Geometry: final body of the model. Coordinates: model frame, mm. Face numbers are marked on the shaded views. A direction names the side the tool comes from. Give positions to 0.01 mm unless a question says otherwise; leave off trailing zeros. Write each loop counter-clockwise with the first axis right and the second up, starting at its lowest first coordinate (ties: lowest second). Pieces come first, ordered by that corner, then holes. Notation, with made-up numbers: M 60.5,54 L 71.5,54 A8 cw 71.5,69 Z; hole C 36.25,-33 d8. An arc over 180 degrees is marked long. Answer as a JSON object with one key per item and string values.
from build123d import *

# Parameters (mm, degrees)
SKETCH1_R           = 50.8
SKETCH1_W           = 38.0365
SKETCH1_H           = 12.7508
BOSS_EXTRUDE1_DEPTH = 5.6642
SKETCH1_3_R         = 50.8
SKETCH1_3_W         = 38.0365
SKETCH1_3_H         = 12.7508
SKETCH1_3_R_2       = 3.71475
BOSS_EXTRUDE2_DEPTH = 5.715
BOSS_EXTRUDE3_DEPTH = 15.875
CUT_EXTRUDE1_DEPTH  = 22.5392


with BuildPart() as part:
    # Sketch1 → Boss-Extrude1 (new body)
    with BuildSketch(Plane(origin=(0, 0, 0), x_dir=(1, 0, 0), z_dir=(0, 1, 0))):
        Circle(SKETCH1_R)
        Rectangle(SKETCH1_W, SKETCH1_H, mode=Mode.SUBTRACT)
    extrude(amount=BOSS_EXTRUDE1_DEPTH)

    # Sketch1_3 → Boss-Extrude2 (add)
    with BuildSketch(Plane(origin=(0, 0, 0), x_dir=(1, 0, 0), z_dir=(0, 1, 0))):
        Circle(SKETCH1_3_R)
        Rectangle(SKETCH1_3_W, SKETCH1_3_H, mode=Mode.SUBTRACT)
        Rectangle(SKETCH1_3_W, SKETCH1_3_H)
        Circle(SKETCH1_3_R_2, mode=Mode.SUBTRACT)
    extrude(amount=-BOSS_EXTRUDE2_DEPTH)

    # Sketch2 → Boss-Extrude3 (add, symmetric)
    with BuildSketch(Plane(origin=(0, 0, 0), x_dir=(1, 0, 0), z_dir=(0, 1, 0))):
        with BuildLine():
            Line((-32.174984, 35.112833), (-34.319983, 37.453689))
            ThreePointArc((-34.319983, 37.453689), (0, 50.8), (34.319983, 37.453689))
            Line((34.319983, 37.453689), (32.174984, 35.112833))
            ThreePointArc((32.174984, 35.112833), (0, 47.625), (-32.174984, 35.112833))
        make_face()
        with BuildLine():
            Line((-25.588894, -40.166518), (-27.29482, -42.844285))
            ThreePointArc((-27.29482, -42.844285), (0, -50.8), (27.29482, -42.844285))
            Line((27.29482, -42.844285), (25.588894, -40.166518))
            ThreePointArc((25.588894, -40.166518), (0, -47.625), (-25.588894, -40.166518))
        make_face()
    extrude(amount=BOSS_EXTRUDE3_DEPTH, both=True)

    # Sketch3 → Cut-Extrude1 (cut, through all)
    with BuildSketch(Plane(origin=(0, 5.6642, 0), x_dir=(1, 0, 0), z_dir=(0, 1, 0))):
        with BuildLine():
            Line((-31.75, 17.8054), (31.75, 17.8054))
            ThreePointArc((31.75, 17.8054), (0, 33.0454), (-31.75, 17.8054))
        make_face()
        with BuildLine():
            Line((-31.75, -17.8054), (31.75, -17.8054))
            ThreePointArc((31.75, -17.8054), (0, -33.0454), (-31.75, -17.8054))
        make_face()
    extrude(amount=-CUT_EXTRUDE1_DEPTH, mode=Mode.SUBTRACT)


solid = part.part
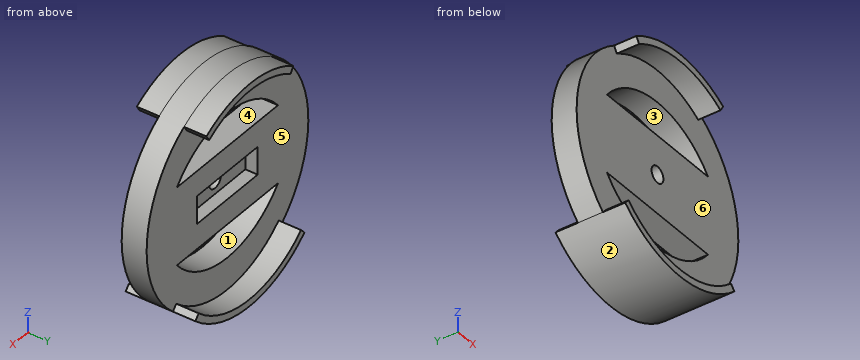
1) Set-up query: the marked faces 4, 5 and 6. Return all of +Z, -Z, +X, -X, +Y, -Y with unobstructed straight access to the full face (end or side cutting, diameter ignored); none if empty.
Geometry check:
{"face 4": "+Y, -Y", "face 5": "+Y", "face 6": "-Y"}
2) Cut plane A-A on y = 7.5. Return loops of the section in (x, z) (3 decimals).
Geometry check:
{"outline": "M -34.32,-37.454 A50.8 ccw 34.32,-37.454 L 32.175,-35.113 A47.625 cw -32.175,-35.113 Z; M -27.295,42.844 L -25.589,40.167 A47.625 cw 25.589,40.167 L 27.295,42.844 A50.8 ccw Z"}
3) Line query: line 1 (X direction, y = -2.2, z = 0); line 2 (Y direction, x = 11.5, z = 3.5) (3 decimals); line 3 (Y direction, x = 21, z = -30) (3 decimals). Output: solid intervals per line, ascending. Write a range as from..to.
Geometry check:
{"line 1": "x = -50.8..-3.71, 3.71..50.8", "line 2": "y = -5.715..0", "line 3": "y = -5.715..5.664"}
4) Cut plane D-D on y = -3. Return loops of the section in (x, z), and give its area (3 significant figures).
Geometry check:
{"outline": "M -34.32,-37.45 A50.8 ccw 34.32,-37.45 A50.8 ccw long Z; hole M -31.75,-17.81 A40.69 ccw 31.75,-17.81 Z; hole M -31.75,17.81 L 31.75,17.81 A40.69 ccw Z; hole C 0,0 d7.43", "area": "6,720 mm2"}
5) Cut plane B-B on z = -23.5. Return loops of the section in (x, y) (3 decimals).
Geometry check:
{"outline": "M -45.038,-5.715 L -26.187,-5.715 L -26.187,5.664 L -45.038,5.664 Z; M 26.187,-5.715 L 45.038,-5.715 L 45.038,5.664 L 26.187,5.664 Z"}
6) Contact query for flat-ended pins moving along their axis: P1, Ø1.5, axis at x = -35.5, y = 8.5, coming from the -Z side; P2, Ø2, axis at x = 31.5, y = 2, coming from the +Z side (3 decimals); P3, Ø12.5, axis at x = -11, y = 2, coming from the -Z side; P4, Ø1.7, axis at x = -6.5, y = 2.5, coming from the -Z side. Output: stop coordinate, or through.
Geometry check:
{"P1": "passes through", "P2": "stops at z = 40.625", "P3": "stops at z = -50.58", "P4": "stops at z = -50.48"}
7) Cut plane C-C on x = -17.5. Return loops of the section in (y, z) (3 decimals), and give its area (3 significant figures).
Geometry check:
{"outline": "M -15.875,-47.691 L 15.875,-47.691 L 15.875,-44.293 L 5.664,-44.293 L 5.664,-29.09 L -5.715,-29.09 L -5.715,-44.293 L -15.875,-44.293 Z; M -15.875,44.293 L -5.715,44.293 L -5.715,29.09 L 5.664,29.09 L 5.664,44.293 L 15.875,44.293 L 15.875,47.691 L -15.875,47.691 Z; M -5.715,-17.805 L 5.664,-17.805 L 5.664,-6.375 L 0,-6.375 L 0,6.375 L 5.664,6.375 L 5.664,17.805 L -5.715,17.805 Z", "area": "895 mm2"}
8) Pull-direction query (Z, two-part tool) for the marked faces 1, 2 and 3; classes: pulls with the +Z half, pulls with the -Z half, needs draft (parallel to the pull), parting line crosses it, or undercut.
Geometry check:
{"face 1": "undercut", "face 2": "pulls with the -Z half", "face 3": "undercut"}
